from build123d import *

# Parameters (mm, degrees)
F0_R      = 28.475
F1_DEPTH  = 12
F2_W      = 19.991411
F2_H      = 4
F3_DEPTH  = 25
F4_R      = 1.5
F5_DEPTH  = 25
F7_DEPTH  = 3
F8_W      = 12.31
F8_H      = 4.5
F9_DEPTH  = 3.5
F10_W     = 12.31
F10_H     = 24
F11_DEPTH = 25
F12_R     = 1
F13_DEPTH = 25


with BuildPart() as f1:
    # F0 (on Front) → F1 (new body)
    with BuildSketch(Plane.XZ):
        with BuildLine():
            ThreePointArc((29.171904, -7), (29.792257, -3.524406), (30, 0))
            ThreePointArc((30, 0), (29.792257, 3.524406), (29.171904, 7))
            ThreePointArc((29.171904, 7), (-30, 0), (29.171904, -7))
        make_face()
        Circle(F0_R, mode=Mode.SUBTRACT)
        with BuildLine():
            Line((39, 0), (30, 0))
            ThreePointArc((30, 0), (29.792257, -3.524406), (29.171904, -7))
            Line((29.171904, -7), (39, -7))
            Line((39, -7), (39, 0))
        make_face()
        with BuildLine():
            ThreePointArc((29.171904, 7), (29.792257, 3.524406), (30, 0))
            Line((30, 0), (39, 0))
            Line((39, 0), (39, 7))
            Line((39, 7), (29.171904, 7))
        make_face()
    extrude(amount=F1_DEPTH)

    # F2 (on face) → F3 (cut)
    with BuildSketch(Plane.XZ.offset(12)):
        with Locations((34.155282, 0)):
            Rectangle(F2_W, F2_H)
    extrude(amount=-F3_DEPTH, mode=Mode.SUBTRACT)

    # F4 (on face) → F5 (cut)
    with BuildSketch(Plane(origin=(0, 0, -7), x_dir=(1, 0, 0), z_dir=(0, 0, -1))):
        with Locations((34.085952, 6)):
            Circle(F4_R)
    extrude(amount=-F5_DEPTH, mode=Mode.SUBTRACT)

    # F6 (on face) → F7 (join)
    with BuildSketch(Plane.XZ.offset(12)):
        with BuildLine():
            Line((-43, 16.5), (-43, 0))
            Line((-43, 0), (-43, -16.5))
            Line((-43, -16.5), (-25.05494, -16.5))
            Line((-25.05494, -16.5), (-23.207232, -16.5))
            ThreePointArc((-23.207232, -16.5), (-28.595733, 0), (-23.207232, 16.5))
            Line((-23.207232, 16.5), (-25.05494, 16.5))
            Line((-25.05494, 16.5), (-43, 16.5))
        make_face()
    extrude(amount=-F7_DEPTH)

    # F8 (on face) → F9 (join)
    with BuildSketch(Plane.XZ.offset(12)):
        with Locations((-36.845, 14.25)):
            Rectangle(F8_W, F8_H)
        with Locations((-36.845, -14.25)):
            Rectangle(F8_W, F8_H)
    extrude(amount=F9_DEPTH)

    # F10 (on face) → F11 (cut)
    with BuildSketch(Plane.XZ.offset(12)):
        with Locations((-36.845, 0)):
            Rectangle(F10_W, F10_H)
    extrude(amount=-F11_DEPTH, mode=Mode.SUBTRACT)

    # F12 (on face) → F13 (cut)
    with BuildSketch(Plane(origin=(0, -9, 0), x_dir=(-1, 0, 0), z_dir=(0, 1, 0))):
        with Locations((36.845, 14.25)):
            Circle(F12_R)
        with Locations((36.845, -14.25)):
            Circle(F12_R)
    extrude(amount=-F13_DEPTH, mode=Mode.SUBTRACT)


solid = f1.part
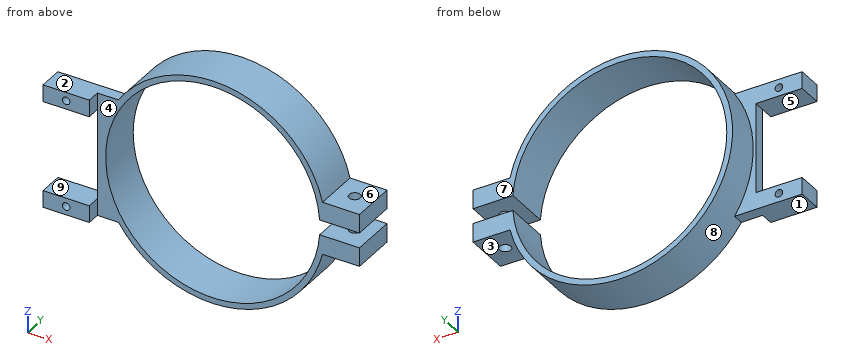
Build history of the part. All positions in model axes, mm. Face numbers are marked on the shaded views. A direction names the side the tool comes from. Give positions to 0.01 mm unless a question says otherwise; leave off trailing zeros. Order: outer loops, then holes, each group sorted by start corner. A loop starts at its lowest first (then second) coordinate and runs counter-clockwise, first axis right, second up. Notation, with made-up numbers: M -38,-4.5 L -33,-4.5 A18 cw -33,21.5 Z; hole C 65,52 d6. An arc over 180 degrees is marked long. Put each result on its own line as item: value.
Item 1: Which spindle directions (+Z, -Z, +X, -X, +Y, -Y) get a long thin tool onto all of the face, cutting with end or side? Do the marked faces 1, 2, 3, 4 and 5. Say none if no direction does.
Results are:
face 1: -Z, -X, +Y, -Y
face 2: +Z, -X, +Y, -Y
face 3: -Z, +X, +Y, -Y
face 4: +Z, -Z, +X, -Y
face 5: -X, +Y, -Y
Item 2: Cut at B-B on y = -10.25. Write the cut outline in (x, z) (3 decimals), then the cut area to 3 significant figures.
Results are:
outline: M -43,-16.5 L -25.055,-16.5 A30 ccw 29.172,-7 L 39,-7 L 39,-2 L 28.405,-2 A28.475 cw long 28.405,2 L 39,2 L 39,7 L 29.172,7 A30 ccw -25.055,16.5 L -43,16.5 L -43,12 L -30.69,12 L -30.69,-12 L -43,-12 Z; hole C -36.845,-14.25 d2; hole C -36.845,14.25 d2
area: 548 mm2
Item 3: Cut at A-A on x = 0. Write the cut outline in (y, z) (3 decimals).
Results are:
outline: M -12,-30 L 0,-30 L 0,-28.475 L -12,-28.475 Z; M -12,28.475 L 0,28.475 L 0,30 L -12,30 Z
Item 4: Cut at C-C on z = -14.25. Write the cut outline in (x, y) (3 decimals).
Results are:
outline: M -43,-15.5 L -37.845,-15.5 L -37.845,-9 L -43,-9 Z; M -35.845,-15.5 L -30.69,-15.5 L -30.69,-12 L -24.653,-12 L -24.653,0 L -26.4,0 L -26.4,-9 L -35.845,-9 Z; M 24.653,-12 L 26.4,-12 L 26.4,0 L 24.653,0 Z
Item 5: Drop flat-ended pins along their axis: pin 1 Ø7 at (x, y) = (-36, -13.5) entering from +Z; pin 2 Ø1.8 at (x, z) = (-36.845, -14.25) entering from +Y; pin 3 Ø3 at (x, y) = (-40, -13.5) entering from -Z; pin 4 Ø3 at (y, z) = (-14, -14.5) entering from +X. Give the stop position or say it passes through.
Results are:
pin 1: z = 16.5
pin 2: through
pin 3: z = -16.5
pin 4: x = -30.69
Item 6: Wall check: probe 1 along Z at (x, y) = (32, -10.75); probe 2 along X at (y, z) = (-6, 4.25); probe 3 along X at (y, z) = (-5.75, -5.5). Give the ranges that are in metal, low to high.
Results are:
probe 1: -7 to -2, 2 to 7
probe 2: -29.7 to -28.16, 28.16 to 32.59, 35.59 to 39
probe 3: -29.49 to -27.94, 27.94 to 32.61, 35.56 to 39
Item 7: Pull direction Z, two halves, no side cores. Call the marked faces 6, 7, 8 and 9: +Z half, -Z half, draft (parallel to the pull), parting line (faces both ways), or undercut.
Results are:
face 6: +Z half
face 7: draft
face 8: parting line
face 9: undercut
Item 8: Cut at D-D on z = 10.5. Write the cut outline in (x, y), then the cut area to 3 significant figures.
Results are:
outline: M -30.69,-12 L -26.47,-12 L -26.47,0 L -28.1,0 L -28.1,-9 L -30.69,-9 Z; M 26.47,-12 L 28.1,-12 L 28.1,0 L 26.47,0 Z
area: 47.0 mm2
